from build123d import *

# Parameters (mm, degrees)
F1_DEPTH  = 2
F2_W      = 2
F2_H      = 18.4
F2_H_2    = 13
F2_H_3    = 10
F3_DEPTH  = 4
F2_R      = 1.25
F4_DEPTH  = 4
F2_R_2    = 2
F5_DEPTH  = 2.4
F6_DEPTH  = 15.5
F7_R      = 3.5
F7_R_2    = 1
F8_DEPTH  = 32
F10_DEPTH = 28
F11_R     = 0.875
F12_DEPTH = 10
F14_DEPTH = 25
F16_DEPTH = 1


with BuildPart() as f1:
    # F0 (on Top) → F1 (new body)
    with BuildSketch(Plane.XY):
        with BuildLine():
            Line((-50.909091, 30), (-50.909091, -30))
            ThreePointArc((-50.909091, -30), (59.090909, 0), (-50.909091, 30))
        make_face()
    extrude(amount=F1_DEPTH)

    # F2 (on face) → F3 (join)
    with BuildSketch(Plane.XY.offset(2)):
        with BuildLine():
            ThreePointArc((-48.909091, 29.449495), (57.090909, 0), (-48.909091, -29.449495))
            Line((-48.909091, -29.449495), (-48.909091, -22.050505))
            Line((-48.909091, -22.050505), (-50.909091, -22.050505))
            Line((-50.909091, -22.050505), (-50.909091, -30))
            ThreePointArc((-50.909091, -30), (59.090909, 0), (-50.909091, 30))
            Line((-50.909091, 30), (-50.909091, 19.349495))
            Line((-50.909091, 19.349495), (-48.909091, 19.349495))
            Line((-48.909091, 19.349495), (-48.909091, 29.449495))
        make_face()
        with Locations((-49.909091, -2.850505)):
            Rectangle(F2_W, F2_H)
        with Locations((-49.909091, 12.849495)):
            Rectangle(F2_W, F2_H_2)
        with Locations((-49.909091, -17.050505)):
            Rectangle(F2_W, F2_H_3)
    extrude(amount=F3_DEPTH)

    # F2 (on face) → F4 (join)
    with BuildSketch(Plane.XY.offset(2)):
        with Locations((-33.609091, 25.949495)):
            Circle(F2_R)
        with Locations((-34.909091, -22.350505)):
            Circle(F2_R)
        with Locations((17.190909, 10.749495)):
            Circle(F2_R)
        with Locations((17.190909, -17.150505)):
            Circle(F2_R)
    extrude(amount=F4_DEPTH)

    # F2 (on face) → F5 (join)
    with BuildSketch(Plane.XY.offset(2)):
        with Locations((-33.609091, 25.949495)):
            Circle(F2_R_2)
        with Locations((-33.609091, 25.949495)):
            Circle(F2_R, mode=Mode.SUBTRACT)
        with Locations((-34.909091, -22.350505)):
            Circle(F2_R_2)
        with Locations((-34.909091, -22.350505)):
            Circle(F2_R, mode=Mode.SUBTRACT)
        with Locations((17.190909, -17.150505)):
            Circle(F2_R_2)
        with Locations((17.190909, -17.150505)):
            Circle(F2_R, mode=Mode.SUBTRACT)
        with Locations((17.190909, 10.749495)):
            Circle(F2_R_2)
        with Locations((17.190909, 10.749495)):
            Circle(F2_R, mode=Mode.SUBTRACT)
    extrude(amount=F5_DEPTH)

    # F2 (on face) → F6 (join)
    with BuildSketch(Plane.XY.offset(2)):
        with BuildLine():
            ThreePointArc((-48.909091, 29.449495), (57.090909, 0), (-48.909091, -29.449495))
            Line((-48.909091, -29.449495), (-48.909091, -22.050505))
            Line((-48.909091, -22.050505), (-50.909091, -22.050505))
            Line((-50.909091, -22.050505), (-50.909091, -30))
            ThreePointArc((-50.909091, -30), (59.090909, 0), (-50.909091, 30))
            Line((-50.909091, 30), (-50.909091, 19.349495))
            Line((-50.909091, 19.349495), (-48.909091, 19.349495))
            Line((-48.909091, 19.349495), (-48.909091, 29.449495))
        make_face()
        with Locations((-49.909091, -2.850505)):
            Rectangle(F2_W, F2_H)
    extrude(amount=F6_DEPTH)

    # F7 (on face) → F8 (join)
    with BuildSketch(Plane.XY.offset(2)):
        with Locations((0, 50.090909)):
            Circle(F7_R)
        with Locations((0, 50.090909)):
            Circle(F7_R_2, mode=Mode.SUBTRACT)
        with Locations((50.090909, 0)):
            Circle(F7_R)
        with Locations((50.090909, 0)):
            Circle(F7_R_2, mode=Mode.SUBTRACT)
        with Locations((0, -50.090909)):
            Circle(F7_R)
        with Locations((0, -50.090909)):
            Circle(F7_R_2, mode=Mode.SUBTRACT)
    extrude(amount=F8_DEPTH)

    # F9 (on face) → F10 (join)
    with BuildSketch(Plane.XY.offset(2)):
        with BuildLine():
            Line((42.607181, 38), (21.590909, 38))
            Line((21.590909, 38), (21.590909, 30.5))
            Line((21.590909, 30.5), (42.590909, 30.5))
            Line((42.590909, 30.5), (42.590909, -10.5))
            Line((42.590909, -10.5), (21.590909, -10.5))
            Line((21.590909, -10.5), (21.590909, -18))
            Line((21.590909, -18), (43.590909, -18))
            Line((43.590909, -18), (43.590909, 36.867391))
            ThreePointArc((43.590909, 36.867391), (43.102766, 37.436927), (42.607181, 38))
        make_face()
    extrude(amount=F10_DEPTH)

    # F11 (on face) → F12 (cut)
    with BuildSketch(Plane.XY.offset(30)):
        with Locations((27.090909, 34)):
            Circle(F11_R)
        with Locations((37.090909, 34)):
            Circle(F11_R)
        with Locations((27.090909, -14)):
            Circle(F11_R)
        with Locations((37.090909, -14)):
            Circle(F11_R)
    extrude(amount=-F12_DEPTH, mode=Mode.SUBTRACT)

    # F13 (on face) → F14 (cut)
    with BuildSketch(Plane.XZ.offset(18)):
        Polygon((34.090909, 30), (30.090909, 30), (30.090909, 23), (28.090909, 21), (28.090909, 2), (36.090909, 2), (36.090909, 21), (34.090909, 23), align=None)
    extrude(amount=-F14_DEPTH, mode=Mode.SUBTRACT)

    # F15 (on face) → F16 (join)
    with BuildSketch(Plane.XY.offset(17.5)):
        with BuildLine():
            Line((-50.909091, -28.185925), (-50.909091, -30))
            ThreePointArc((-50.909091, -30), (59.090909, 0), (-50.909091, 30))
            Line((-50.909091, 30), (-50.909091, 28.185925))
            ThreePointArc((-50.909091, 28.185925), (58.190909, 0), (-50.909091, -28.185925))
        make_face()
    extrude(amount=F16_DEPTH)


solid = f1.part
Geometry: final body of the model. Coordinates: model frame, mm. A direction names the side the tool comes from. Round coordinates to 2 decimals unless told otherwise and drop trailing zeros. Order: outer loops, then holes, each group sorted by start corner. A loop starts at its lowest first (then second) coordinate and runs counter-clockwise, first axis right, second up. Notation, with made-up numbers: (58.5, 75) -> (81.5, 75) arc R11 cw to (81.5, 90) -> close; hole circle Ø7 at (43.25, 60.25). An arc over 180 degrees is marked (long way). Put each result on its own line as item: value. Start each with the question number.
Q1. Reachability of faces 4 (the flat face through (26, -14, 30)), 5 (the cylindrical face through (-32.417, 26.325, 5.189)) from +Z, -Z, +X, -X, +Y, -Y: full face, straight path, thin tool, end or side. Return the list, or none.
Q2. Section B-B on x = -8. Return the cut outline in (y, z).
Q3. Line query: probe 1 along Y at (x, z) = (0, 8.25); probe 2 along Y at (x, z) = (35.5, 11); probe 3 along X at (y, z) = (-2, 12). Output: solid intervals per line, ascending.
Q4. Section C-C on y = 16. Return the cut outline in (x, z), and give its area (3 significant figures).
Q5. Section A-A on z = 14. Give the number of separate pieces and of enclosed holes in the cut face, and give its area (3 significant figures).
Q6. First-contact query: pin 1 (2 mm diameter, centred on x = -50, z = 14, fed in from +Y); pin 2 (3 mm diameter, centred on x = 16.5, y = 11, fed in from +Z); pin 3 (5 mm diameter, centred on x = -20, y = 21.5, fed in from +Z). Flat tips, straight axial feed; report the tip coordinate or a pass-through.
Q7. Section D-D on x = -30. Return the cut outline in (y, z), and give its area (3 significant figures).
Q8. Pull-direction query (Y, two-part tool) for faces 1 (the flat face through (36.091, -14, 11)), 2 (the cylindrical face through (59.05, -2.16, 9.12)), 3 (the flat face through (3, 1, 0)); classes: +Y half, -Y half, draft (parallel to the pull), parting line (faces both ways), or undercut.
Ans:
1. face 4: +Z, +X, -X, +Y, -Y
1. face 5: +Z
2. outline: (-58.55, 0) -> (58.55, 0) -> (58.55, 18.5) -> (57.64, 18.5) -> (57.64, 17.5) -> (56.53, 17.5) -> (56.53, 2) -> (-56.53, 2) -> (-56.53, 17.5) -> (-57.64, 17.5) -> (-57.64, 18.5) -> (-58.55, 18.5) -> close
3. probe 1: y = -59.09 to -57.09, -53.59 to -51.09, -49.09 to -46.59, 46.59 to 49.09, 51.09 to 53.59, 57.09 to 59.09
3. probe 2: y = -47.24 to -44.71, 30.5 to 38, 44.71 to 47.24
3. probe 3: x = -50.91 to -48.91, 42.59 to 43.59, 47.22 to 52.96, 57.06 to 59.06
4. outline: (-50.91, 0) -> (56.88, 0) -> (56.88, 18.5) -> (55.95, 18.5) -> (55.95, 17.5) -> (54.8, 17.5) -> (54.8, 2) -> (43.59, 2) -> (43.59, 30) -> (42.59, 30) -> (42.59, 2) -> (-48.91, 2) -> (-48.91, 6) -> (-50.91, 6) -> close
4. area: 285 mm2
5. separate pieces: 6
5. enclosed holes: 3
5. area: 1,090 mm2
6. pin 1: stops at y = 33.03
6. pin 2: stops at z = 6
6. pin 3: stops at z = 2
7. outline: (-50.91, 0) -> (50.91, 0) -> (50.91, 18.5) -> (49.86, 18.5) -> (49.86, 17.5) -> (48.57, 17.5) -> (48.57, 2) -> (-48.57, 2) -> (-48.57, 17.5) -> (-49.86, 17.5) -> (-49.86, 18.5) -> (-50.91, 18.5) -> close
7. area: 278 mm2
8. face 1: undercut
8. face 2: parting line
8. face 3: draft
